Can you work these out from the model? Positions are in its coordinate system, mm. A direction names the side the tool comes from. Round coordinates to 2 decimals unless told otherwise and drop trailing zeros. Loops run counter-clockwise (first coordinate to the right, second up) from the corner with the lowest first, then second, coordinate; pieces in that order, holes last. Notation, with made-up numbers: (-24, 66.25) -> (27, 66.25) arc R27 cw to (27, 99.25) -> close; hole circle Ø9 at (33, 6). An arc over 180 degrees is marked (long way). Write each question's results on one line, items separated by ' | '.
from build123d import *

# Parameters (mm, degrees)
F0_R     = 4.75
F0_R_2   = 2.75
F1_DEPTH = 7
F2_R     = 1.540286
F3_DEPTH = 7


with BuildPart() as f1:
    # F0 (on Top) → F1 (new body)
    with BuildSketch(Plane.XY):
        Circle(F0_R)
        Circle(F0_R_2, mode=Mode.SUBTRACT)
    extrude(amount=F1_DEPTH)

    # F2 (on Front) → F3 (join)
    with BuildSketch(Plane.XZ):
        with Locations((0, 3.492086)):
            Circle(F2_R)
    extrude(amount=F3_DEPTH)


solid = f1.part
1. If we section it at A-A (x = 0): List the corners of the cut face in (y, z) for me.
Final values:
outline: (-7, 1.95) -> (-4.75, 1.95) -> (-4.75, 0) -> (-2.75, 0) -> (-2.75, 1.95) -> (0, 1.95) -> (0, 5.03) -> (-2.75, 5.03) -> (-2.75, 7) -> (-4.75, 7) -> (-4.75, 5.03) -> (-7, 5.03) -> close; (2.75, 0) -> (4.75, 0) -> (4.75, 7) -> (2.75, 7) -> close
2. Please list where these lines run through material, in increasing order: line 1 (Y direction, x = 0, z = 5.25); line 2 (Y direction, x = 0, z = 3.25); line 3 (X direction, y = 1.25, z = 4). Write a range as from..to.
Final values:
line 1: -4.75..-2.75, 2.75..4.75 | line 2: -7..0, 2.75..4.75 | line 3: -4.58..-2.45, 2.45..4.58
3. We'd pull the mould along Y, two halves only. Please class faces 3 (the face through (0, -3, 0)), 4 (the face through (0, 0, 4)), 5 (the face through (1.47, -1.36, 3.95)), 6 (the face through (0, -7, 4)): pulls with the +Y half, pulls with the -Y half, needs draft (parallel to the pull), parting line crosses it, or undercut.
Final values:
face 3: needs draft | face 4: undercut | face 5: undercut | face 6: pulls with the -Y half
4. On a 3-axis mill with a long thin cutter (end or side, diameter ignored), from which of +Z, -Z, +X, -X, +Y, -Y can I reach the whole of each face in a straight line? I mean faces 1 (the face through (-0.334, -5.726, 1.988)), 2 (the face through (0, -3, 7)). Say none if no direction works.
Final values:
face 1: -Y | face 2: +Z, +X, -X, +Y, -Y
5. Will these pins go through, and if not, where does the flat tip stop? pin 1 (2 mm diameter, centred on x = 2.5, z = 5, fed in from -Y); pin 2 (1 mm diameter, centred on x = 3, z = 1, fed in from +Y); pin 3 (4.5 mm diameter, centred on x = 0, y = 0, fed in from -Z).
Final values:
pin 1: y = -4.51 | pin 2: y = 4.04 | pin 3: z = 1.95
6. If we section it at B-B (y = -0.25): List the corners of the cut face in (x, z) for me.
Final values:
outline: (-4.74, 0) -> (-2.74, 0) -> (-2.74, 7) -> (-4.74, 7) -> close; circle Ø3.08 at (0, 3.49); (2.74, 0) -> (4.74, 0) -> (4.74, 7) -> (2.74, 7) -> close
7. If we section it at C-C (z = 2.75): List the corners of the cut face in (x, y) for me, then the cut area to 3 significant figures.
Final values:
outline: (-1.35, -7) -> (1.35, -7) -> (1.35, -4.55) arc R4.75 ccw (long way) to (-1.35, -4.55) -> close; hole (-1.35, -2.4) -> (-1.35, 0) -> (1.35, 0) -> (1.35, -2.4) arc R2.75 ccw (long way) to start | area: 60.5 mm2
8. If we section it at D-D (y = -2): List the corners of the cut face in (x, z) for me, then the cut area to 3 significant figures.
Final values:
outline: (-4.31, 0) -> (-1.89, 0) -> (-1.89, 7) -> (-4.31, 7) -> close; circle Ø3.08 at (0, 3.49); (1.89, 0) -> (4.31, 0) -> (4.31, 7) -> (1.89, 7) -> close | area: 41.3 mm2
